Here's how the part is built. I have some questions about the finished solid (model axes, mm). Face numbers are marked on the shaded views. A direction names the side the tool comes from. Round coordinates to 2 decimals unless told otherwise and drop trailing zeros. Loops run counter-clockwise (first coordinate to the right, second up) from the corner with the lowest first, then second, coordinate; pieces in that order, holes last. Notation, with made-up numbers: M -6.75,17 L 47.25,17 A20 ccw 47.25,40 Z; hole C -12,50.25 d7. An arc over 180 degrees is marked long. Write item = value, one per line. Start each with the question number.
from build123d import *

# Parameters (mm, degrees)
SM_BASE_FLANGE_1_DEPTH = 3.1
SKETCH_11_W            = 1.15
SKETCH_11_H            = 0.4
SKETCH_13_W            = 1.15
SKETCH_13_H            = 0.4
SKETCH_15_W            = 1.712954878
SKETCH_15_H            = 1
EXTRUDE_1_DEPTH        = 0.4
FILLET_1_R             = 0.25


# Sheet-metal steps are written as plain solids
with BuildPart() as part:
    # Sketch 1 → 基体-法兰1 (new body)
    with BuildSketch(Plane.XY):
        with BuildLine():
            Line((0, 8), (0.283974596, 7.83604719))
            ThreePointArc((0.283974596, 7.83604719), (0.749900423, 7.228840832), (0.65, 6.470021787))
            Line((0.65, 6.470021787), (0.288675135, 5.844188762))
            ThreePointArc((0.288675135, 5.844188762), (0.154700538, 5.344188762), (0.288675135, 4.844188762))
            Line((0.288675135, 4.844188762), (0.861324865, 3.852330333))
            ThreePointArc((0.861324865, 3.852330333), (0.995299462, 3.352330333), (0.861324865, 2.852330333))
            Line((0.861324865, 2.852330333), (0.133974596, 1.592522712))
            ThreePointArc((0.133974596, 1.592522712), (0.034074174, 1.351341757), (0, 1.092522712))
            Line((0, 1.092522712), (0, 0.7366))
            ThreePointArc((0, 0.7366), (0.215745145, 0.215745145), (0.7366, 0))
            Line((0.7366, 0), (3.2634, 0))
            ThreePointArc((3.2634, 0), (3.784254855, 0.215745145), (4, 0.7366))
            Line((4, 0.7366), (4, 1.092522712))
            ThreePointArc((4, 1.092522712), (3.965925826, 1.351341757), (3.866025404, 1.592522712))
            Line((3.866025404, 1.592522712), (3.138675135, 2.852330333))
            ThreePointArc((3.138675135, 2.852330333), (3.004700538, 3.352330333), (3.138675135, 3.852330333))
            Line((3.138675135, 3.852330333), (3.711324865, 4.844188762))
            ThreePointArc((3.711324865, 4.844188762), (3.845299462, 5.344188762), (3.711324865, 5.844188762))
            Line((3.711324865, 5.844188762), (3.35, 6.470021787))
            ThreePointArc((3.35, 6.470021787), (3.250099577, 7.228840832), (3.716025404, 7.83604719))
            Line((3.716025404, 7.83604719), (4, 8))
            Line((4, 8), (4.2, 7.653589838))
            Line((4.2, 7.653589838), (3.916025404, 7.489637029))
            ThreePointArc((3.916025404, 7.489637029), (3.636469908, 7.125313214), (3.696410162, 6.670021787))
            Line((3.696410162, 6.670021787), (4.057735027, 6.044188762))
            ThreePointArc((4.057735027, 6.044188762), (4.245299462, 5.344188762), (4.057735027, 4.644188762))
            Line((4.057735027, 4.644188762), (3.485085296, 3.652330333))
            ThreePointArc((3.485085296, 3.652330333), (3.404700538, 3.352330333), (3.485085296, 3.052330333))
            Line((3.485085296, 3.052330333), (4.212435565, 1.792522712))
            ThreePointArc((4.212435565, 1.792522712), (4.352296157, 1.454869375), (4.4, 1.092522712))
            Line((4.4, 1.092522712), (4.4, 0.7366))
            ThreePointArc((4.4, 0.7366), (4.067097567, -0.067097567), (3.2634, -0.4))
            Line((3.2634, -0.4), (0.7366, -0.4))
            ThreePointArc((0.7366, -0.4), (-0.067097567, -0.067097567), (-0.4, 0.7366))
            Line((-0.4, 0.7366), (-0.4, 1.092522712))
            ThreePointArc((-0.4, 1.092522712), (-0.352296157, 1.454869375), (-0.212435565, 1.792522712))
            Line((-0.212435565, 1.792522712), (0.514914704, 3.052330333))
            ThreePointArc((0.514914704, 3.052330333), (0.595299462, 3.352330333), (0.514914704, 3.652330333))
            Line((0.514914704, 3.652330333), (-0.057735027, 4.644188762))
            ThreePointArc((-0.057735027, 4.644188762), (-0.245299462, 5.344188762), (-0.057735027, 6.044188762))
            Line((-0.057735027, 6.044188762), (0.303589838, 6.670021787))
            ThreePointArc((0.303589838, 6.670021787), (0.363530092, 7.125313214), (0.083974596, 7.489637029))
            Line((0.083974596, 7.489637029), (-0.2, 7.653589838))
            Line((-0.2, 7.653589838), (0, 8))
        make_face()
    extrude(amount=SM_BASE_FLANGE_1_DEPTH)

    # 扫描1: sweep along a path in 草图12
    with BuildLine(Plane(origin=(2, 0, 0), x_dir=(0, 0, -1), z_dir=(1, 0, 0))) as sweep_1_path:
        Line((-3.5, -3.6), (-3.5, -0.4))
        ThreePointArc((-3.5, -0.4), (-3.441421356, -0.258578644), (-3.3, -0.2))
        Line((-3.3, -0.2), (-3.1, -0.2))
    # 草图11 → 扫描1 (sweep)
    with BuildSketch(Plane.XY.offset(3.1)):
        with Locations((2, -0.2)):
            Rectangle(SKETCH_11_W, SKETCH_11_H)
    sweep(path=sweep_1_path.line)

    # 扫描2: sweep along a path in 草图14
    with BuildLine(Plane(origin=(2, 0, 0), x_dir=(0, 0, -1), z_dir=(1, 0, 0))) as sweep_2_path:
        Line((0, -0.2), (0.2, -0.2))
        ThreePointArc((0.2, -0.2), (0.341421356, -0.258578644), (0.4, -0.4))
        Line((0.4, -0.4), (0.4, -3.4))
    # 草图13 → 扫描2 (sweep)
    with BuildSketch(Plane(origin=(0, 0, 0), x_dir=(-1, 0, 0), z_dir=(0, 0, -1))):
        with Locations((-2, -0.2)):
            Rectangle(SKETCH_13_W, SKETCH_13_H)
    sweep(path=sweep_2_path.line)

    # 草图15 → 凸台-拉伸1 (add)
    with BuildSketch(Plane(origin=(0, 0, 0), x_dir=(-1, 0, 0), z_dir=(0, 0, -1))):
        with Locations((-0.710838396, 5.344188762)):
            Rectangle(SKETCH_15_W, SKETCH_15_H)
    extrude(amount=EXTRUDE_1_DEPTH)

    # 圆角1
    fillet_1_edges = [part.edges().sort_by_distance(p)[0] for p in [
        (-0.145639043, 4.844188762, -0.2),
        (-0.145639043, 5.844188762, -0.2),
        (-0.145639043, 5.344188762, -0.4),
    ]]
    fillet(fillet_1_edges, radius=FILLET_1_R)


solid = part.part
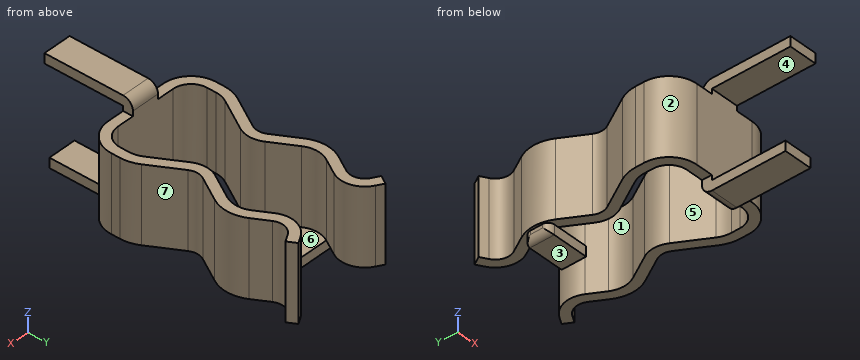
Item 1: I want a section at B-B, the plane y = -2.5. List the corners of the cut face in (x, z) for me (3 decimals).
Item 2: Please list where these lines run through material, in increasing order: line 1 (X direction, y = 7, z = 1.3); line 2 (X direction, y = 1, z = 1.8); line 3 (Y direction, x = 1.8, z = 0.65). Write a range as [from, to].
Item 3: I want a section at A-A, the plane x = 1.2. List the corners of the cut face in (y, z) for me.
Item 4: We'd pull the mould along Y, two halves only. Please class the marked faces 1, 2 and 3: released by +Y, released by -Y, zero draft, split by the parting line, or undercut.
Item 5: For the marked faces 4, 5, 6 and 7, which set-ups out of +Z, -Z, +X, -X, +Y, -Y let a thin tool reach every point of the face, with its end or its side?
Item 6: Will these pins go through, and if not, where does the flat tip stop? pin 1 Ø2 at (x, y) = (2.5, 3) entering from +Z; pin 2 Ø2 at (x, y) = (4, 4.5) entering from -Z; pin 3 Ø0.7 at (y, z) = (-2, -0.5) entering from +X (3 decimals).
Worked out:
q1.outline = M 1.425,-0.6 L 2.575,-0.6 L 2.575,-0.2 L 1.425,-0.2 Z; M 1.425,3.3 L 2.575,3.3 L 2.575,3.7 L 1.425,3.7 Z
q2.line_1 = [0.38, 0.78], [3.22, 3.62]
q2.line_2 = [-0.4, 0], [4, 4.4]
q2.line_3 = [-0.4, 0]
q3.outline = M -0.4,0 L 0,0 L 0,3.1 L -0.4,3.1 Z; M 4.84,-0.4 L 5.84,-0.4 L 5.84,0 L 4.84,0 Z
q4.face_1 = undercut
q4.face_2 = released by -Y
q4.face_3 = zero draft
q5.face_4 = +X, -X, -Y
q5.face_5 = +Z, -Z
q5.face_6 = +Z
q5.face_7 = +Z, -Z, +X
q6.pin_1 = 3.1
q6.pin_2 = 0
q6.pin_3 = 2.575
